Here's the drawing with two shaded views (mm, measured from the low corner). I have some questions. Give positions to 0.01 mm unless a question says otherwise; leave off trailing zeros. Loops run counter-clockwise (first coordinate to the right, second up) from the corner with the lowest first, then second, coordinate; pieces in that order, holes last. Notation, with made-up numbers: (-27, -20) - (-7, -20) arc R10 cw to (-7, -4) - close; hole circle Ø10 at (-21, 46). An arc over 180 degrees is marked (long way). Answer as a JSON object with one key per item and string values. Group by question number.
Item 1: Please list where these lines run through material, in increasing order: L1, parallel to X at y = 7.5, z = 8; L2, parallel to Z at x = 55.75, y = 8.25; L3, parallel to Y at x = 16, z = 9.75.
Item 2: Will these pins go through, and if not, where does the flat tip stop? pin 1 (12 mm diameter, centred on x = 35.75, y = 77, fed in from +Z); pin 2 (4 mm diameter, centred on x = 15.5, z = 6, fed in from -Y).
Item 3: Suppose I cut it at D-D on x = 15.75. Write out the boundary of the cut face in (y, z), and give its area (3 significant figures).
Item 4: Suppose I cut it at B-B on z = 6.75. Write out the boundary of the cut face in (x, y).
Item 5: Thinking about a two-plate mould opening in Y: for the marked faces 1, 2 and 3, which applies, pulls with the +Y half, pulls with the -Y half, needs draft (parallel to the pull), parting line crosses it, or undercut?
Item 6: Suppose I cut it at C-C on y = 77. Write out the boundary of the cut face in (x, z), and give its area (3 significant figures).
Item 7: Suppose I cut it at A-A on x = 35.75. Write out the boundary of the cut face in (y, z), and give its area (3 significant figures).
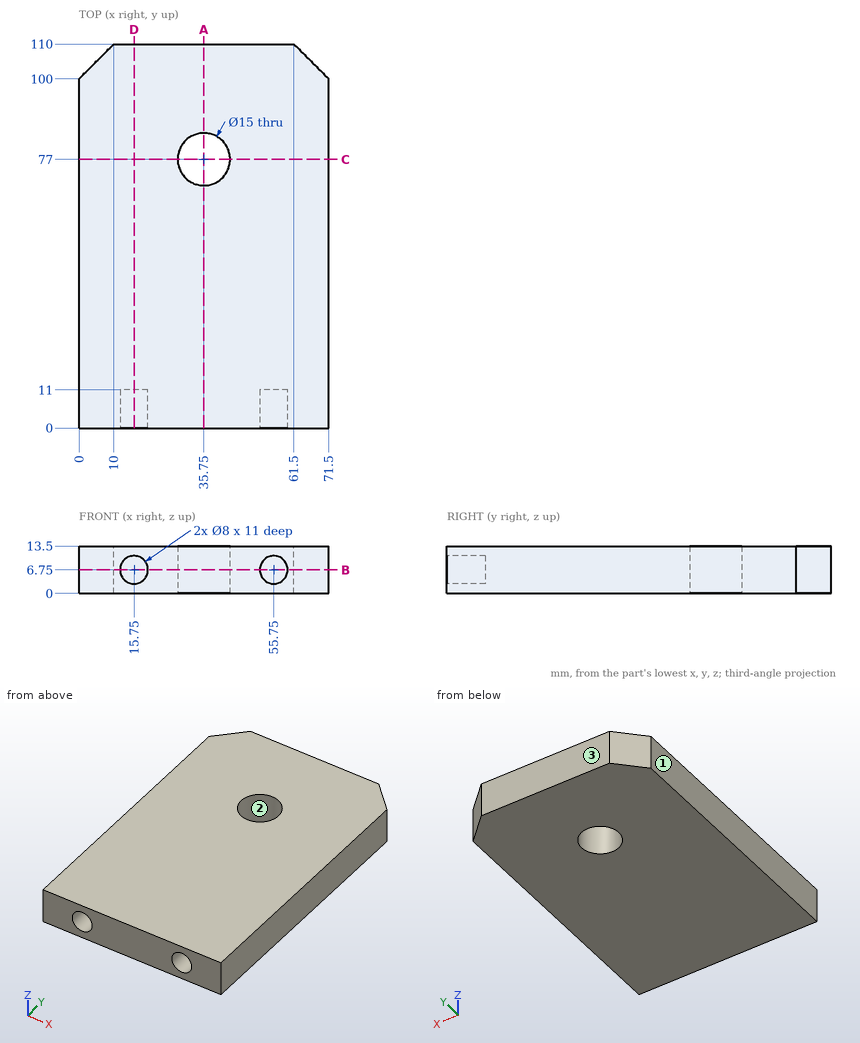
Worked out:
{
 "1": {"L1": "x = 0 to 11.95, 19.55 to 51.95, 59.55 to 71.5", "L2": "z = 0 to 2.75, 10.75 to 13.5", "L3": "y = 11 to 110"},
 "2": {"pin 1": "passes through", "pin 2": "stops at y = 11"},
 "3": {"outline": "(0, 0) - (110, 0) - (110, 13.5) - (0, 13.5) - (0, 10.75) - (11, 10.75) - (11, 2.75) - (0, 2.75) - close", "area": "1,400 mm2"},
 "4": {"outline": "(0, 0) - (11.75, 0) - (11.75, 11) - (19.75, 11) - (19.75, 0) - (51.75, 0) - (51.75, 11) - (59.75, 11) - (59.75, 0) - (71.5, 0) - (71.5, 100) - (61.5, 110) - (10, 110) - (0, 100) - close; hole circle Ø15 at (35.75, 77)"},
 "5": {"face 1": "needs draft", "face 2": "undercut", "face 3": "pulls with the +Y half"},
 "6": {"outline": "(0, 0) - (28.25, 0) - (28.25, 13.5) - (0, 13.5) - close; (43.25, 0) - (71.5, 0) - (71.5, 13.5) - (43.25, 13.5) - close", "area": "763 mm2"},
 "7": {"outline": "(0, 0) - (69.5, 0) - (69.5, 13.5) - (0, 13.5) - close; (84.5, 0) - (110, 0) - (110, 13.5) - (84.5, 13.5) - close", "area": "1,280 mm2"}
}
